Could you check a few things on this model? Use its own coordinates, in mm. A direction names the side the tool comes from. Coordinates: 2 decimals unless noted, no trailing zeros. Write each loop counter-clockwise with the first axis right and the second up, starting at its lowest first coordinate (ties: lowest second). Pieces come first, ordered by that corner, then holes. Notation, with made-up numbers: M 89.5,46.25 L 117.5,46.25 A19 ccw 117.5,65.25 Z; hole C 13.25,49 d10. An arc over 180 degrees is marked long. Write item = value, one per line.
```python
from build123d import *

# Parameters (mm, degrees)
F0_W      = 60.4223795235
F0_H      = 126.5786588192
F0_W_2    = 4.2580850422
F0_H_2    = 11.6458535194
F1_DEPTH  = 12.7
F4_DEPTH  = 25
F5_W      = 44.0693465061
F5_H      = 24.1423398256
F6_DEPTH  = 25
F7_W      = 27.9744537547
F7_H      = 6.1313877814
F8_DEPTH  = 25
F10_DEPTH = 25
F13_DEPTH = 150


with BuildPart() as f1:
    # F0 (on Top) → F1 (new body, symmetric)
    with BuildSketch(Plane.XY):
        with Locations((4.1334796697, 0)):
            Rectangle(F0_W, F0_H)
        with Locations((-20.6351820379, 32.8994877636)):
            Rectangle(F0_W_2, F0_H_2, mode=Mode.SUBTRACT)
    extrude(amount=F1_DEPTH, both=True)

    # F3 (on face) → F4 (join)
    with BuildSketch(Plane.XY.offset(12.7)):
        Polygon((9.2804457981, 43.4682284111), (5.0971903838, 44.1307909787), (0.9139349695, 43.4682284111), (-2.8598342584, 41.545396949), (-5.8547144745, 38.5505167329), (-7.7775459366, 34.776747505), (-8.4401085041, 30.5934920907), (-7.7775459366, 26.4102366764), (-5.8547144745, 22.6364674485), (-2.8598342584, 19.6415872324), (0.9139349695, 17.7187557703), (5.0971903838, 17.0561932027), (9.2804457981, 17.7187557703), (13.054215026, 19.6415872324), (16.0490952421, 22.6364674485), (17.9719267043, 26.4102366764), (18.6344892718, 30.5934920907), (17.9719267043, 34.776747505), (16.0490952421, 38.5505167329), (13.054215026, 41.545396949), align=None)
        Polygon((-2.2527005044, 26.4659842643), (5.197609196, 39.0224382281), (12.3466624599, 26.2920537797), align=None, mode=Mode.SUBTRACT)
    extrude(amount=F4_DEPTH)

    # F5 (on face) → F6 (join)
    with BuildSketch(Plane.XY.offset(12.7)):
        with Locations((3.4489056561, -32.3813892901)):
            Rectangle(F5_W, F5_H)
    extrude(amount=F6_DEPTH)

    # F7 (on Top) → F8 (join)
    with BuildSketch(Plane.XY):
        with Locations((6.1313877814, -8.0474459101)):
            Rectangle(F7_W, F7_H)
    extrude(amount=F8_DEPTH)

    # F9 (on face) → F10 (join)
    with BuildSketch(Plane.XY.offset(12.7)):
        with BuildLine():
            add(Edge.make_bspline(
                [(-3.6654782741, -5.0642236167), (-1.2137473257, -5.8734401187), (0.1916065812, -4.7901463695)],
                knots=[5.6666909862, 5.6666909862, 5.6666909862, 6.2831853072, 6.2831853072, 6.2831853072], degree=2, weights=[1, 0.9528668255, 1]))
            add(Edge.make_bspline(
                [(0.1916065812, -4.7901463695), (6.4545371904, 0.0375298105), (-5.1250907994, 10.7039809585)],
                knots=[0, 0, 0, 1.9137670292, 1.9137670292, 1.9137670292], degree=2, weights=[1, 0.5760701954, 1]))
            add(Edge.make_bspline(
                [(-5.1250907994, 10.7039809585), (-9.1468374458, 5.3420650054), (-3.6654782741, -5.0642236167)],
                knots=[0.1210246027, 0.1210246027, 0.1210246027, 1.1768049687, 1.1768049687, 1.1768049687], degree=2, weights=[1, 0.8638717322, 1]))
        make_face()
        with BuildLine():
            add(Edge.make_bspline(
                [(0.1916065812, -4.7901463695), (6.4545371904, 0.0375298105), (-5.1250907994, 10.7039809585)],
                knots=[0, 0, 0, 1.9137670292, 1.9137670292, 1.9137670292], degree=2, weights=[1, 0.5760701954, 1]))
            add(Edge.make_bspline(
                [(-3.6654782741, -5.0642236167), (-1.2137473257, -5.8734401187), (0.1916065812, -4.7901463695)],
                knots=[5.6666909862, 5.6666909862, 5.6666909862, 6.2831853072, 6.2831853072, 6.2831853072], degree=2, weights=[1, 0.9528668255, 1]))
            add(Edge.make_bspline(
                [(-3.6654782741, -5.0642236167), (7.7967294339, -26.8250748804), (21.3915865986, -22.0091251639), (34.9864437633, -17.1931754474), (18.2025562972, 2.6824818924)],
                knots=[1.1768049687, 1.1768049687, 1.1768049687, 2.9445969746, 2.9445969746, 4.7123889804, 4.7123889804, 4.7123889804], degree=2, weights=[1, 0.6341435153, 1, 0.6341435153, 1]))
            add(Edge.make_bspline(
                [(18.2025562972, 2.6824818924), (2.66192218, 21.0858654459), (-5.1250907994, 10.7039809585)],
                knots=[4.7123889804, 4.7123889804, 4.7123889804, 6.4042099098, 6.4042099098, 6.4042099098], degree=2, weights=[1, 0.6630500062, 1]))
        make_face()
        with BuildLine():
            add(Edge.make_bspline(
                [(-5.1250907994, 10.7039809585), (-9.1468374458, 5.3420650054), (-3.6654782741, -5.0642236167)],
                knots=[0.1210246027, 0.1210246027, 0.1210246027, 1.1768049687, 1.1768049687, 1.1768049687], degree=2, weights=[1, 0.8638717322, 1]))
            add(Edge.make_bspline(
                [(-5.1250907994, 10.7039809585), (-16.2578023137, 20.958759749), (-15.2138378826, 9.6808045144), (-14.1698734514, -1.5971507202), (-3.6654782741, -5.0642236167)],
                knots=[1.9137670292, 1.9137670292, 1.9137670292, 3.7902290077, 3.7902290077, 5.6666909862, 5.6666909862, 5.6666909862], degree=2, weights=[1, 0.5912156804, 1, 0.5912156804, 1]))
        make_face()
    extrude(amount=F10_DEPTH)

    # F12 (on face) + F10_face (on face) → F13 (join)
    with BuildSketch(Plane.XY.offset(12.7)):
        Polygon((-15.1200483821, 58.7558450371), (-4.268118646, 54.9524389207), (-3.0674270983, 48.5890431418), (6.9253058173, 54.9524389207), (6.3772096892, 67.5610487277), (-4.8162147741, 73.3906884605), (-15.4615431093, 66.6117183864), align=None)
        Polygon((-3.0674270983, 48.5890431418), (-4.268118646, 54.9524389207), (-15.1200483821, 58.7558450371), (-14.9134469812, 54.0031085795), (-3.7200225179, 48.1734688466), align=None)
        Polygon((-1.6542957296, 41.0997639807), (-3.0674270983, 48.5890431418), (-3.7200225179, 48.1734688466), (-14.9134469812, 54.0031085795), (-15.1200483821, 58.7558450371), (-17.5717985126, 59.6151393441), (-28.2616554628, 50.4251648275), (-25.6478325464, 36.5724898875), (-12.3441526798, 31.9097894641), align=None)
        Polygon((28.3961594105, 33.5202328861), (21.9387635589, 52.3932985961), (3.0656978488, 45.9359027445), (8.3079936012, 30.6142166531), (14.9058774114, 30.8326855302), (14.9690065658, 28.9261493169), align=None)
        Polygon((15.9268081188, 0), (14.9690065658, 28.9261493169), (9.5230937004, 27.0628370345), (8.3079936012, 30.6142166531), (-15.9268081188, 29.8117548227), (-14.9058774114, -1.0209307075), align=None)
        Polygon((9.5230937004, 27.0628370345), (14.9690065658, 28.9261493169), (14.9058774114, 30.8326855302), (8.3079936012, 30.6142166531), align=None)
    with BuildSketch(Plane(origin=(4.9113998877, -19.1714286629, 37.7), x_dir=(1, 0, 0), z_dir=(0, 0, 1))):
        with BuildLine():
            Line((20.5721790215, -25.2811305401), (20.5721790215, -1.1387907144))
            Line((20.5721790215, -1.1387907144), (19.0393327914, -1.1387907144))
            add(Edge.make_bspline(
                [(19.0393327914, -1.1387907144), (21.2490059306, 1.3356954103), (22.1859609961, 5.7952845742), (20.4843675369, 11.8248238632), (16.8415372864, 17.6495119094), (9.1694693906, 26.7348559867), (2.9158744634, 32.08683227), (-3.618455925, 34.3337423373), (-7.9712190855, 32.6288930507), (-10.0364906871, 29.8754096213)],
                knots=[3.2381563984, 3.2381563984, 3.2381563984, 3.2381563984, 3.2381563984, 3.2381563984, 4.7123889804, 4.7123889804, 4.7123889804, 4.7123889804, 6.4238462878, 6.4238462878, 6.4238462878, 6.4238462878, 6.4238462878, 6.4238462878], degree=5, weights=[0.9897321171, 0.9732134667, 0.9503985365, 0.9627650148, 1, 1, 0.9545858807, 0.9545858807, 1, 1]))
            add(Edge.make_bspline(
                [(-10.0364906871, 29.8754096213), (-21.1692022014, 40.1301884118), (-20.1252377703, 28.8522331772), (-19.0812733391, 17.5742779427), (-8.5768781618, 14.1072050461)],
                knots=[1.9137670292, 1.9137670292, 1.9137670292, 3.7902290077, 3.7902290077, 5.6666909862, 5.6666909862, 5.6666909862], degree=2, weights=[1, 0.5912156804, 1, 0.5912156804, 1]))
            add(Edge.make_bspline(
                [(-8.5768781618, 14.1072050461), (-6.867540918, 10.8620506684), (-4.3486920685, 7.1585507312), (-1.0610908327, 3.5964338438), (2.6377751049, 0.7453286942), (6.2308483777, -1.1387907144)],
                knots=[1.1768049687, 1.1768049687, 1.1768049687, 1.1768049687, 1.1768049687, 1.1768049687, 2.2161101678, 2.2161101678, 2.2161101678, 2.2161101678, 2.2161101678, 2.2161101678], degree=5, weights=[1, 1, 0.9814943061, 0.9662423378, 0.9632109021, 0.968574194]))
            Line((6.2308483777, -1.1387907144), (-23.4971674847, -1.1387907144))
            Line((-23.4971674847, -1.1387907144), (-23.4971674847, -25.2811305401))
            Line((-23.4971674847, -25.2811305401), (20.5721790215, -25.2811305401))
        make_face()
    extrude(amount=F13_DEPTH)


solid = f1.part
```
Item 1: I'm going to push flat-ended pins straight in: P1, Ø22, axis at x = 9, y = 31.5, coming from the +Z side; P2, Ø1, axis at x = -17.5, z = 11.5, coming from the +Y side; P3, Ø1, axis at y = -23.5, z = 153.5, coming from the -X side. Where does each tip first touch, or does it pass through?
Numbers:
P1 = 162.7
P2 = 63.29
P3 = -18.59
Item 2: If we mould it in two halves opening along Y, with no side actions, what happens to faces 6 (the face through (3, -44.453, 99)), 7 (the face through (1.859, 51.726, 86.65)), 8 (the face through (-10.06, 70.05, 86.65))? For each: pulls with the +Y half, pulls with the -Y half, needs draft (parallel to the pull), parting line crosses it, or undercut.
Numbers:
face_6 = pulls with the -Y half
face_7 = undercut
face_8 = pulls with the +Y half
Item 3: Imagine slicing it at A-A (z = 0). Write out the boundary of the cut face in (x, y).
Numbers:
outline = M -26.08,-63.29 L 34.34,-63.29 L 34.34,63.29 L -26.08,63.29 Z; hole M -22.76,27.08 L -18.51,27.08 L -18.51,38.72 L -22.76,38.72 Z
Item 4: If I drill on line 1 along Y through (x, z) = (-7, 143); line 2 along Y through (x, z) = (-7, 29); line 3 along Z through (x, y) = (-10.5, 58), over which ranges is the centre line in solid material (lowest first)?
Numbers:
line_1 = -44.45 to -20.31, -3.27 to 30.11, 36.5 to 72
line_2 = -44.45 to -20.31, -3.27 to 36.3, 36.5 to 72
line_3 = -12.7 to 162.7
Item 5: For faces 1 (the face through (6.655, 61.168, 86.65)), 2 (the face through (25.484, -33, 99)), 3 (the face through (-21, 38.722, 0)), 4 (the face through (17, 24.5, 25)), 5 (the face through (-5, -8, 25)), which set-ups out of +Z, -Z, +X, -X, +Y, -Y let a thin tool reach every point of the face, with its end or its side?
Numbers:
face_1 = +Z, +X, +Y
face_2 = +Z, +X, -Y
face_3 = -Z
face_4 = +Z, +X
face_5 = +Z, -X
Item 6: Imagine slicing it at B-B (y = -40). Write out the boundary of the cut face in (x, z), and give its area (3 significant figures).
Numbers:
outline = M -26.08,-12.7 L 34.34,-12.7 L 34.34,12.7 L 25.48,12.7 L 25.48,187.7 L -18.59,187.7 L -18.59,12.7 L -26.08,12.7 Z
area = 9,250 mm²
